```python
from build123d import *

# Parameters (mm, degrees)
F0_R     = 1
F1_DEPTH = 2.5


with BuildPart() as f1:
    # F0 (on Right) → F1 (new body)
    with BuildSketch(Plane.YZ):
        with BuildLine():
            Line((-15.844449, -1), (15.844449, -1))
            ThreePointArc((15.844449, -1), (17.180755, -1.181879), (18.419842, -1.714286))
            ThreePointArc((18.419842, -1.714286), (21.45, 0), (18.419842, 1.714286))
            ThreePointArc((18.419842, 1.714286), (17.180755, 1.181879), (15.844449, 1))
            Line((15.844449, 1), (-15.844449, 1))
            ThreePointArc((-15.844449, 1), (-17.180755, 1.181879), (-18.419842, 1.714286))
            ThreePointArc((-18.419842, 1.714286), (-21.45, 0), (-18.419842, -1.714286))
            ThreePointArc((-18.419842, -1.714286), (-17.180755, -1.181879), (-15.844449, -1))
        make_face()
        with Locations((-19.45, 0)):
            Circle(F0_R, mode=Mode.SUBTRACT)
        with Locations((19.45, 0)):
            Circle(F0_R, mode=Mode.SUBTRACT)
    extrude(amount=F1_DEPTH)


solid = f1.part
```
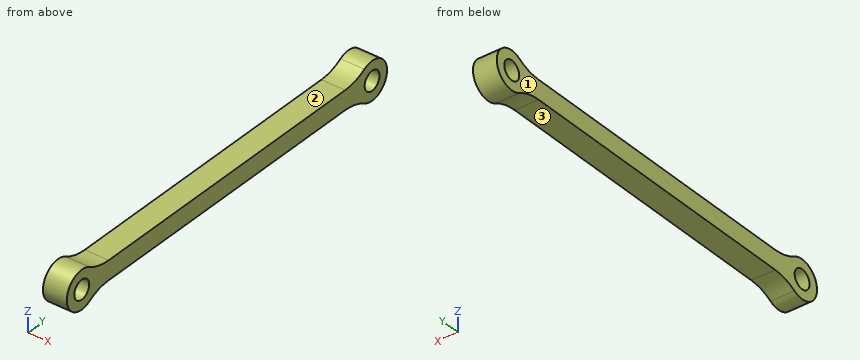
The listing builds one solid part. Answer for the finished solid, in the listing's coordinates (mm). Face numbers are marked on the shaded views. A direction names the side the tool comes from. Round coordinates to 2 decimals unless told otherwise and drop trailing zeros. Order: outer loops, then holes, each group sorted by start corner. A loop starts at its lowest first (then second) coordinate and runs counter-clockwise, first axis right, second up. Notation, with made-up numbers: (5.5, 87) -> (14.5, 87) arc R19 ccw to (14.5, 92) -> close; hole circle Ø4 at (34.5, 53.25). An arc over 180 degrees is marked (long way). Answer as CSV lines item,"result". Start each with the question number.
(1) The part is cut by section D-D (y = 9.5). Determine the outline of the cut face in (x, z).
(2) The part is cut by section A-A (y = 19.45). Determine the outline of the cut face in (x, z).
(3) A flat-ended cylindrical pin translates along its axis: pin 1 Ø1.5 at (x, y) = (2, 3) entering from +Z. Find the tip coordinate at first contact, or state that the pin passes through.
(4) A tool of negligible diameter and unlimited length cuts with its end or side. For the marked faces 1, 2 and 3, from which of +Z, -Z, +X, -X, +Y, -Y can it reach the whole face along a straight path? Write none if from no direction.
(5) The part is cut by section C-C (x = 1.3). Determine the outline of the cut face in (y, z).
(6) The part is cut by section B-B (z = 0). Determine the outline of the cut face in (x, y), then the cut area to 4 significant figures.
(7) Find the intervals of material crossed by probe 1 along Y at (x, z) = (1.25, -0.1); probe 2 along Y at (x, z) = (2.4, 0.8); probe 3 along Z at (x, y) = (1.1, -19.45), in increasing order. Write a range as from..to.
Evaluation:
1,outline,"(0, -1) -> (2.5, -1) -> (2.5, 1) -> (0, 1) -> close"
2,outline,"(0, -2) -> (2.5, -2) -> (2.5, -1) -> (0, -1) -> close; (0, 1) -> (2.5, 1) -> (2.5, 2) -> (0, 2) -> close"
3,pin 1,"z = 1"
4,face 1,"+Z, -Z, -X, +Y, -Y"
4,face 2,"+Z, +X, -X"
4,face 3,"-Z, +X, -X"
5,outline,"(-18.42, -1.71) arc R5 cw to (-15.84, -1) -> (15.84, -1) arc R5 cw to (18.42, -1.71) arc R2 ccw (long way) to (18.42, 1.71) arc R5 cw to (15.84, 1) -> (-15.84, 1) arc R5 cw to (-18.42, 1.71) arc R2 ccw (long way) to start; hole circle Ø2 at (-19.45, 0); hole circle Ø2 at (19.45, 0)"
6,outline,"(0, -21.45) -> (2.5, -21.45) -> (2.5, -20.45) -> (0, -20.45) -> close; (0, -18.45) -> (2.5, -18.45) -> (2.5, 18.45) -> (0, 18.45) -> close; (0, 20.45) -> (2.5, 20.45) -> (2.5, 21.45) -> (0, 21.45) -> close"
6,area,"97.25 mm²"
7,probe 1,"-21.45..-20.44, -18.46..18.46, 20.44..21.45"
7,probe 2,"-21.28..-20.05, -18.85..18.85, 20.05..21.28"
7,probe 3,"-2..-1, 1..2"
